Could you check a few things on this model? Use its own coordinates, in mm. Coordinates: 2 decimals unless noted, no trailing zeros. Write each loop counter-clockwise with the first axis right and the second up, starting at its lowest first coordinate (ties: lowest second). Pieces come first, ordered by that corner, then holes.
Item 1: If I drill on probe 1 along X at (y, z) = (-1028, 2.2); probe 2 along X at (y, z) = (-1119, 1.9); probe 3 along X at (y, z) = (-524, 2.35), over which ranges is the centre line in solid material (lowest first)?
Item 2: Thinking about a two-plate mould opening in Y: for faces 1 (the cylindrical face through (72.115, -1067.321, 1.479)), 2 (the flat face through (28, -961, 0)), which applies, +Y half, -Y half, draft (parallel to the pull), parting line (faces both ways), or undercut?
Item 3: I want a section at B-B on y = -739. Please give me the cut outline in (x, z).
Item 4: For P1, Ø8, axis at x = 8, y = -839, coming from the +Z side, with a flat end and sliding along its axis, tell me the tip position at first contact or that it passes through.
Item 5: I want a section at A-A on z = 0.6. State how many separate pieces and enclosed holes the cut face has, then the cut area to 3 significant figures.
Autodesk Inventor part; units mm, degrees
ref_plane "YZ Plane" through (0, 0, 0) normal (1, 0, 0) x (0, 1, 0)
ref_plane "XZ Plane" through (0, 0, 0) normal (0, 1, 0) x (-1, 0, 0)
ref_plane "XY Plane" through (0, 0, 0) normal (0, 0, 1) x (1, 0, 0)
sketch "Sketch1" plane through (0, 0, 0) normal (0, 0, 1) x (1, 0, 0)
  line L0 (0, 100) -> (0, 50) construction
  line L1 (0, 47) -> (0, 0) construction
  line L2 (0, 50) -> (0, 47) construction
  arc A0 (38, -1950) -> (19, 0) centre (-10977.8747, -1082.2416) ccw
  line L3 (38, -1950) -> (0, -1950)
  line L4 (0, -1950) -> (0, 0)
  line L5 (0, 0) -> (19, 0)
  line L6 (14.9159, 0) -> (33.6838, -210)
  line L7 (33.6838, -210) -> (37.5713, -209.058)
  dimension "d115" = 3
  dimension "d131" = 11050
  dimension "d132" = 19
  dimension "d133" = 38
  dimension "d134" = 1950
  dimension "d145" = 4
  dimension "d146" = 210
extrude "Plate3" add sketch "Sketch1" along normal blind 3 contours L3 L4 L5 L6 L7 A0
sketch "Sketch3" plane through (0, 0, 0) normal (0, 0, -1) x (-1, 0, 0)
  line L0 (0, 0) -> (0, -1950)
  line L1 (-14.9159, 0) -> (0, 0)
  arc A0 (-37.5713, -209.058) -> (-38, -1950) centre (10977.8747, -1082.2416) ccw
  line L2 (0, -1950) -> (-38, -1950)
  circle A1 centre (-8, -1910) radius 3.5
  circle A2 centre (0, -1907.1277) radius 5
  circle A3 centre (0, -1907.1277) radius 12
  line L3 (-33.6838, -210) -> (-14.9159, 0)
  line L4 (-37.5713, -209.058) -> (-33.6838, -210)
  point P0 (0, -1895.1277)
  point P1 (-11.2941, -1911.1827)
  point P2 (-4.7059, -1908.8173)
  point P3 (0, -1902.1277)
  dimension "d135" = 7
  dimension "d136" = 8
  dimension "d137" = 40
  dimension "d143" = 10
extrude "Extrusion2" cut sketch "Sketch3" against normal blind 10 contours A1
pattern_linear "Rectangular Pattern1" count 31 spacing 63 along (0, 1, 0) of "Extrusion2"
equation "\"BendReliefWidth\" = Thickness"
equation "\"BendReliefDepth\" = 0.5 * Thickness"
equation "\"CornerReliefSize\" = 4 * Thickness"
equation "\"MinimumRemnant\" = 2 * Thickness"
equation "\"GapSize\" = Thickness"
properties part number "MSC 079 creen pillar" material "AISI304"
Response values:
1. probe 1: x = 0 to 4.5, 11.5 to 71.99
1. probe 2: x = 0 to 72.06
1. probe 3: x = 0 to 4.5, 11.5 to 58.02
2. face 1: parting line
2. face 2: draft
3. outline: (0, 0) - (66.79, 0) - (66.79, 3) - (0, 3) - close
4. P1: stops at z = 3
5. separate pieces: 1
5. enclosed holes: 31
5. area: 110,000 mm2
